Could you check a few things on this model? Use its own coordinates, in mm. Face numbers are marked on the shaded views. A direction names the side the tool comes from. Round coordinates to 2 decimals unless told otherwise and drop trailing zeros. Write each loop counter-clockwise with the first axis right and the second up, starting at its lowest first coordinate (ties: lowest second). Pieces come first, ordered by that corner, then holes. Notation, with made-up numbers: (-9.75, 24) -> (10.25, 24) arc R28 cw to (10.25, 47) -> close; hole circle Ø9 at (23, 3.5). An arc over 180 degrees is marked (long way). One line per question, with ' | ' between items. Start each with the question number.
1. For pin 1 Ø2.5 at (x, z) = (0.5, -1) entering from -Y; pin 2 Ø2 at (x, y) = (-0.5, 6.5) entering from -Z; pin 3 Ø2 at (x, y) = (-0.5, 7.5) entering from +Z, each with a flat end and sliding along its axis, tell me the tip position at first contact or that it passes through.
2. Thinking about a two-plate mould opening in Z: for the marked faces 1, 2 and 3, which applies, released by +Z, released by -Z, zero draft, split by the parting line, or undercut?
3. Imagine slicing it at B-B, the plane z = 0. List the corners of the cut face in (x, y) for me, and give its area (3 significant figures).
4. For the marked faces 4, 5 and 6, which set-ups out of +Z, -Z, +X, -X, +Y, -Y let a thin tool reach every point of the face, with its end or its side?
5. Imagine slicing it at A-A, the plane x = 0. List the corners of the cut face in (y, z) for me, and give its area (3 significant figures).
6. If I drill on line 1 along Z through (x, y) = (-0.15, 0.75); line 2 along Y through (x, z) = (-0.15, -1.7), over which ranges is the centre line in solid material (lowest first)? Write a range as [from, to].
7. Imagine slicing it at D-D, the plane y = 6.75. List the corners of the cut face in (x, z) for me.
8. Imagine slicing it at C-C, the plane y = 0.75. List the corners of the cut face in (x, z) for me, and give its area (3 significant figures).
Autodesk Inventor part; units mm, degrees
ref_plane "YZ Plane" through (0, 0, 0) normal (1, 0, 0) x (0, 1, 0)
ref_plane "XZ Plane" through (0, 0, 0) normal (0, 1, 0) x (-1, 0, 0)
ref_plane "XY Plane" through (0, 0, 0) normal (0, 0, 1) x (1, 0, 0)
sketch "Sketch1" plane through (0, 0, 0) normal (0, 1, 0) x (-1, 0, 0)
  line L0 (-2.3495, 2.3495) -> (2.3495, 2.3495)
  line L1 (2.3495, 2.3495) -> (2.3495, -2.3495)
  line L2 (2.3495, -2.3495) -> (-2.3495, -2.3495)
  line L3 (-2.3495, -2.3495) -> (-2.3495, 2.3495)
  line L4 (-2.3495, 2.3495) -> (2.3495, -2.3495) construction
  line L5 (2.3495, 2.3495) -> (-2.3495, -2.3495) construction
  point P0 (0, 0)
  dimension "d0" = 4.699
  dimension "width" = 4.699
extrude "Extrusion1" add sketch "Sketch1" along normal blind 2.667
sketch "Sketch2" plane through (0, 2.667, 0) normal (0, 1, 0) x (1, 0, 0)
  circle A0 centre (0, 0) radius 1.4986
  dimension "d4" = 2.9972
extrude "Extrusion2" add sketch "Sketch2" along normal blind 6.223
sketch "Sketch3" plane through (0, 0, 0) normal (0, -1, 0) x (1, 0, 0)
  line L0 (-1.778, 1.778) -> (1.778, 1.778)
  line L1 (1.778, 1.778) -> (1.778, -1.778)
  line L2 (1.778, -1.778) -> (-1.778, -1.778)
  line L3 (-1.778, -1.778) -> (-1.778, 1.778)
  line L4 (-1.778, 1.778) -> (1.778, -1.778) construction
  line L5 (1.778, 1.778) -> (-1.778, -1.778) construction
  point P0 (0, 0)
  dimension "d7" = 3.556
  dimension "d8" = 3.556
extrude "Extrusion3" cut sketch "Sketch3" against normal blind 2.159
sketch "Sketch4" plane through (0, 0, 0) normal (0, -1, 0) x (1, 0, 0)
  circle A0 centre (-2.032, 2.032) radius 0.2921
  circle A1 centre (2.032, -2.032) radius 0.2921
  point P0 (0, 0)
  point P1 (0, 0)
  dimension "d11" = 0.5842
  dimension "d12" = 2.032
  dimension "d13" = 2.032
  dimension "d16" = 360
extrude "Extrusion4" add sketch "Sketch4" along normal blind 1.524
equation "\"d0\" = width"
properties part number "VLP-350-F" material "Polycarbonate, Clear"
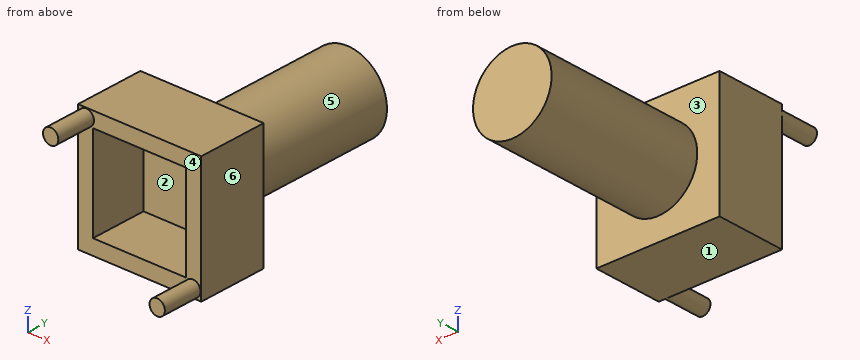
Geometry results:
1) pin 1: stops at y = 0 | pin 2: stops at z = -1.5 | pin 3: stops at z = 1.5
2) face 1: released by -Z | face 2: undercut | face 3: zero draft
3) outline: (-2.35, 0) -> (-1.78, 0) -> (-1.78, 2.16) -> (1.78, 2.16) -> (1.78, 0) -> (2.35, 0) -> (2.35, 2.67) -> (1.5, 2.67) -> (1.5, 8.89) -> (-1.5, 8.89) -> (-1.5, 2.67) -> (-2.35, 2.67) -> close | area: 23.5 mm2
4) face 4: -Y | face 5: +Y | face 6: +Z, -Z, +X, +Y, -Y
5) outline: (0, -2.35) -> (2.67, -2.35) -> (2.67, -1.5) -> (8.89, -1.5) -> (8.89, 1.5) -> (2.67, 1.5) -> (2.67, 2.35) -> (0, 2.35) -> (0, 1.78) -> (2.16, 1.78) -> (2.16, -1.78) -> (0, -1.78) -> close | area: 23.5 mm2
6) line 1: z = [-2.35, -1.78], [1.78, 2.35] | line 2: y = [2.16, 2.67]
7) outline: circle Ø3 at (0, 0)
8) outline: (-2.35, -2.35) -> (2.35, -2.35) -> (2.35, 2.35) -> (-2.35, 2.35) -> close; hole (-1.78, -1.78) -> (1.78, -1.78) -> (1.78, 1.78) -> (-1.78, 1.78) -> close | area: 9.44 mm2
